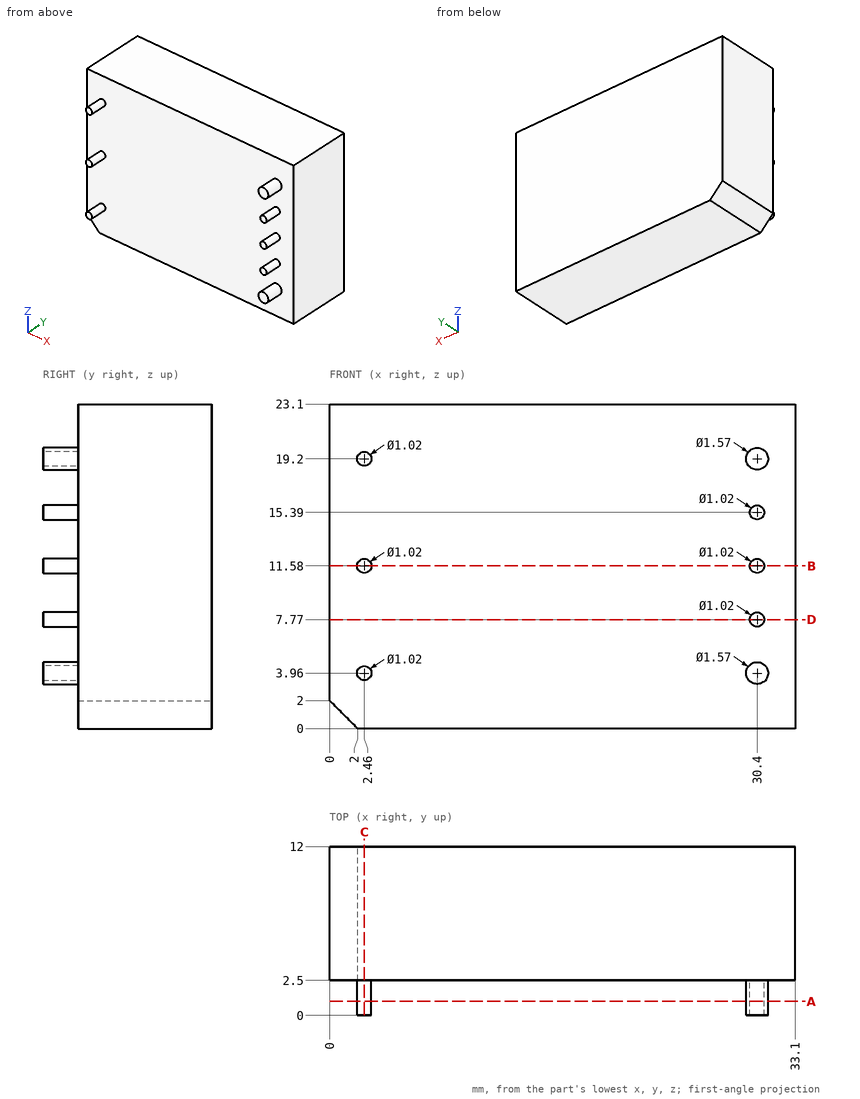
Source: three-view drawing plus pictorial views. Frame: mm from the lowest corner of the part. Coordinates: 2 decimals unless noted, no trailing zeros. Loops run counter-clockwise (first coordinate to the right, second up) from the corner with the lowest first, then second, coordinate; pieces in that order, holes last. Notation, with made-up numbers: (-10, 40.5) - (45, 40.5) arc R17 ccw to (45, 53.5) - close; hole circle Ø1 at (22.5, 43). An arc over 180 degrees is marked (long way). One line per question, with ' | ' between items.
1) Section C-C, the plane x = 2.46. Return loops of the section in (y, z).
Report:
outline: (0, 3.45) - (2.5, 3.45) - (2.5, 0) - (12, 0) - (12, 23.1) - (2.5, 23.1) - (2.5, 19.71) - (0, 19.71) - (0, 18.69) - (2.5, 18.69) - (2.5, 12.09) - (0, 12.09) - (0, 11.07) - (2.5, 11.07) - (2.5, 4.47) - (0, 4.47) - close
2) First-contact query: P1, Ø1.5, axis at x = 13.5, y = 6.5, coming from the -Z side; P2, Ø1.5, axis at x = 27.5, z = 16.5, coming from the -Y side. Flat tips, straight axial feed; report the tip coordinate or a pass-through.
Report:
P1: stops at z = 0 | P2: stops at y = 2.5
3) Section A-A, the plane y = 1. Return loops of the section in (x, z) (3 decimals).
Report:
outline: circle Ø1.02 at (2.46, 3.96); circle Ø1.02 at (2.46, 11.58); circle Ø1.02 at (2.46, 19.2); circle Ø1.57 at (30.4, 3.96); circle Ø1.57 at (30.4, 19.2); circle Ø1.02 at (30.4, 7.77); circle Ø1.02 at (30.4, 11.58); circle Ø1.02 at (30.4, 15.39)
4) Section D-D, the plane z = 7.77. Return loops of the section in (x, y), then the cut area to 3 significant figures.
Report:
outline: (0, 2.5) - (29.89, 2.5) - (29.89, 0) - (30.91, 0) - (30.91, 2.5) - (33.1, 2.5) - (33.1, 12) - (0, 12) - close | area: 317 mm²
5) Line query: line 1 along Y through (x, z) = (28.5, 11.25). Output: solid intervals per line, ascending.
Report:
line 1: y = 2.5 to 12
6) Section B-B, the plane z = 11.58. Return loops of the section in (x, y), then the cut area to 3 significant figures.
Report:
outline: (0, 2.5) - (1.95, 2.5) - (1.95, 0) - (2.97, 0) - (2.97, 2.5) - (29.89, 2.5) - (29.89, 0) - (30.91, 0) - (30.91, 2.5) - (33.1, 2.5) - (33.1, 12) - (0, 12) - close | area: 320 mm²
